Build history of the part. All positions in model axes, mm. A direction names the side the tool comes from. Round coordinates to 2 decimals unless told otherwise and drop trailing zeros. Write each loop counter-clockwise with the first axis right and the second up, starting at its lowest first coordinate (ties: lowest second). Pieces come first, ordered by that corner, then holes. Notation, with made-up numbers: (37, -9.75) -> (89, -9.75) arc R21 ccw to (89, 28.25) -> close; hole circle Ø10 at (32.5, -24). An arc over 180 degrees is marked (long way). Return JSON: item names as keys, results as strings.
from build123d import *

# Parameters (mm, degrees)
F0_R     = 5.5
F0_W     = 48
F0_H     = 82
F1_DEPTH = 24
F2_DEPTH = 4
F3_R     = 3
F4_R     = 5.5
F5_DEPTH = 4


with BuildPart() as f1:
    # F0 (on Top) → F1 (new body)
    with BuildSketch(Plane.XY):
        with BuildLine():
            Line((-14, 54), (-14, 0))
            ThreePointArc((-14, 0), (-9.899495, -9.899495), (0, -14))
            Line((0, -14), (30, -14))
            Line((30, -14), (30, 68))
            Line((30, 68), (0, 68))
            ThreePointArc((0, 68), (-9.899495, 63.899495), (-14, 54))
        make_face()
        Circle(F0_R, mode=Mode.SUBTRACT)
        with Locations((0, 54)):
            Circle(F0_R, mode=Mode.SUBTRACT)
        with Locations((54, 27)):
            Rectangle(F0_W, F0_H)
        with BuildLine():
            Line((78, 68), (78, -14))
            Line((78, -14), (108, -14))
            ThreePointArc((108, -14), (117.899495, -9.899495), (122, 0))
            Line((122, 0), (122, 54))
            ThreePointArc((122, 54), (117.899495, 63.899495), (108, 68))
            Line((108, 68), (78, 68))
        make_face()
        with Locations((108, 0)):
            Circle(F0_R, mode=Mode.SUBTRACT)
        with Locations((108, 54)):
            Circle(F0_R, mode=Mode.SUBTRACT)
    extrude(amount=-F1_DEPTH)

    # F0 (on Top) → F2 (cut)
    with BuildSketch(Plane.XY):
        with Locations((54, 27)):
            Rectangle(F0_W, F0_H)
    extrude(amount=-F2_DEPTH, mode=Mode.SUBTRACT)

    # F3
    f3_edges = [f1.edges().sort_by_distance(p)[0] for p in [
        (78, 27, -4),
        (30, 27, -4),
    ]]
    fillet(f3_edges, radius=F3_R)

    # F4 (on face) → F5 (cut)
    with BuildSketch(Plane(origin=(0, 0, -24), x_dir=(1, 0, 0), z_dir=(0, 0, -1))):
        with BuildLine():
            Line((24, -68), (24, 14))
            Line((24, 14), (0, 14))
            ThreePointArc((0, 14), (-9.899495, 9.899495), (-14, 0))
            Line((-14, 0), (-14, -54))
            ThreePointArc((-14, -54), (-9.899495, -63.899495), (0, -68))
            Line((0, -68), (24, -68))
        make_face()
        with Locations((0, -54)):
            Circle(F4_R, mode=Mode.SUBTRACT)
        Circle(F4_R, mode=Mode.SUBTRACT)
        with BuildLine():
            Line((108, 14), (84, 14))
            Line((84, 14), (84, -68))
            Line((84, -68), (108, -68))
            ThreePointArc((108, -68), (117.899495, -63.899495), (122, -54))
            Line((122, -54), (122, 0))
            ThreePointArc((122, 0), (117.899495, 9.899495), (108, 14))
        make_face()
        with Locations((108, -54)):
            Circle(F4_R, mode=Mode.SUBTRACT)
        with Locations((108, 0)):
            Circle(F4_R, mode=Mode.SUBTRACT)
    extrude(amount=-F5_DEPTH, mode=Mode.SUBTRACT)


solid = f1.part
Q1. Two-plate mould, pull along X, no slides. Class faces 1 (the flat face through (100, 28, 0)), 2 (the cylindrical face through (102.505, 54.242, -9.86)), 3 (the cylindrical face through (117.8, -10, -9.9)), 4 (the cylindrical face through (30.86, 27.57, -3.1)): +X half, -X half, draft (parallel to the pull), parting line (faces both ways), or undercut.
Verdict:
{"face 1": "draft", "face 2": "undercut", "face 3": "+X half", "face 4": "undercut"}
Q2. Wall check: L1, parallel to Y at x = 108, z = -12; L2, parallel to X at y = 0, z = -15.5; L3, parallel to X at y = 1.5, z = -3.25. Give the ranges that are in metal, low to high.
Verdict:
{"L1": "y = -14 to -5.5, 5.5 to 48.5, 59.5 to 68", "L2": "x = -14 to -5.5, 5.5 to 102.5, 113.5 to 122", "L3": "x = -14 to -5.29, 5.29 to 31.02, 76.98 to 102.71, 113.29 to 122"}
Q3. Saw through at D-D on x = 7.5. List the corners of the cut face in (y, z).
Verdict:
{"outline": "(-14, -20) -> (68, -20) -> (68, 0) -> (-14, 0) -> close"}
Q4. Pin check, flat tips, straight feed: pin 1 Ø19 at (x, y) = (94.5, 33.5) entering from -Z; pin 2 Ø2 at (y, z) = (10, -22) entering from -X; pin 3 Ø4.5 at (y, z) = (9, -21.5) entering from +X; pin 4 Ø2 at (y, z) = (57.5, -10.5) entering from +X (3 decimals). Stop position of each tip, or through.
Verdict:
{"pin 1": "stops at z = -20", "pin 2": "stops at x = 24", "pin 3": "stops at x = 122", "pin 4": "stops at x = 121.775"}
Q5. Saw through at C-C on y = 44. List the corners of the cut face in (x, z), then the cut area to 3 significant figures.
Verdict:
{"outline": "(-14, -20) -> (24, -20) -> (24, -24) -> (84, -24) -> (84, -20) -> (122, -20) -> (122, 0) -> (78, 0) -> (78, -1) arc R3 cw to (75, -4) -> (33, -4) arc R3 cw to (30, -1) -> (30, 0) -> (-14, 0) -> close", "area": "2,770 mm²"}
Q6. 3-axis set-ups, long thin cutter, end or side, ignore diameter. For faces 5 (the cylindrical face through (77.14, 27.57, -3.1)), 6 (the flat face through (24, 28, -22)), 7 (the flat face through (84, 26, -22)): which of +Z, -Z, +X, -X, +Y, -Y reach the whole face in a straight line?
Verdict:
{"face 5": "+Z, +Y, -Y", "face 6": "-Z, -X, +Y, -Y", "face 7": "-Z, +X, +Y, -Y"}
Q7. Saw through at B-B on z = -11.25. List the corners of the cut face in (x, y).
Verdict:
{"outline": "(-14, 0) arc R14 ccw to (0, -14) -> (108, -14) arc R14 ccw to (122, 0) -> (122, 54) arc R14 ccw to (108, 68) -> (0, 68) arc R14 ccw to (-14, 54) -> close; hole circle Ø11 at (0, 0); hole circle Ø11 at (0, 54); hole circle Ø11 at (108, 0); hole circle Ø11 at (108, 54)"}
Q8. Saw through at A-A on y = 55.5. List the corners of the cut face in (x, z), then the cut area to 3 significant figures.
Verdict:
{"outline": "(-13.92, -20) -> (-5.29, -20) -> (-5.29, 0) -> (-13.92, 0) -> close; (5.29, -20) -> (24, -20) -> (24, -24) -> (84, -24) -> (84, -20) -> (102.71, -20) -> (102.71, 0) -> (78, 0) -> (78, -1) arc R3 cw to (75, -4) -> (33, -4) arc R3 cw to (30, -1) -> (30, 0) -> (5.29, 0) -> close; (113.29, -20) -> (121.92, -20) -> (121.92, 0) -> (113.29, 0) -> close", "area": "2,350 mm²"}
